Geometry check sheet. Reference: the model listing, model coordinates, mm. Face numbers are marked on the shaded views. A direction names the side the tool comes from. Coordinates: 2 decimals unless noted, no trailing zeros. Loops run counter-clockwise (first coordinate to the right, second up) from the corner with the lowest first, then second, coordinate; pieces in that order, holes last. Notation, with made-up numbers: (50, 49) -> (89, 49) arc R19 ccw to (89, 57) -> close; hole circle Ø9 at (38, 53). An arc over 180 degrees is marked (long way). Answer as a JSON object with one key per item and string values.
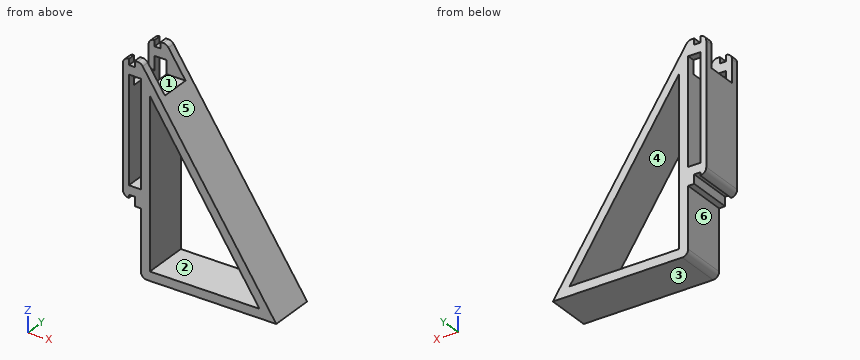
from build123d import *

# Parameters (mm, degrees)
SKETCH2_W               = 4
SKETCH2_H               = 35
BOSS_EXTRUDE1_DEPTH     = 15
CUT_EXTRUDE1_DEPTH      = 87.313382508
CUT_EXTRUDE1_DEPTH_BACK = 15
SKETCH3_W               = 9.5
SKETCH3_H               = 10
FILLET1_R               = 2
FILLET2_R               = 2
FILLET3_R               = 2
FILLET4_R               = 2
FILLET5_R               = 2
FILLET6_R               = 2


with BuildPart() as part:
    # Sketch2 → Boss-Extrude1 (new body)
    with BuildSketch(Plane(origin=(0, 0, 0), x_dir=(1, 0, 0), z_dir=(0, 1, 0))):
        Polygon((0, 0), (0, 2), (2, 2), (2, 0), (4, 0), (49, 68), (4, 68), (4, 46), (2, 46), (2, 43), (0, 43), (0, 44), (-2, 44), (-2, 0), align=None)
        with Locations((2, 22.5)):
            Rectangle(SKETCH2_W, SKETCH2_H, mode=Mode.SUBTRACT)
        Polygon((7, 65), (43.417291153, 65), (7, 9.516238481), align=None, mode=Mode.SUBTRACT)
    extrude(amount=BOSS_EXTRUDE1_DEPTH)

    # Sketch3 → Cut-Extrude1 (cut, two sides: drawn at the far end of the back side and taken through both)
    with BuildSketch(Plane.ZY.offset(2).offset(-CUT_EXTRUDE1_DEPTH_BACK)):
        with Locations((-4.75, 7.5)):
            Rectangle(SKETCH3_W, SKETCH3_H)
    extrude(amount=CUT_EXTRUDE1_DEPTH + CUT_EXTRUDE1_DEPTH_BACK, mode=Mode.SUBTRACT)

    # Fillet1
    fillet1_edges = [part.edges().sort_by_distance(p)[0] for p in [
        (-2, 7.5, -44),
    ]]
    fillet(fillet1_edges, radius=FILLET1_R - 0.0001)  # a hair under: the kernel refuses the full size

    # Fillet2
    fillet2_edges = [part.edges().sort_by_distance(p)[0] for p in [
        (4, 7.5, -68),
    ]]
    fillet(fillet2_edges, radius=FILLET2_R)

    # Fillet3
    fillet3_edges = [part.edges().sort_by_distance(p)[0] for p in [
        (4, 1.25, 0),
    ]]
    fillet(fillet3_edges, radius=FILLET3_R)

    # Fillet4
    fillet4_edges = [part.edges().sort_by_distance(p)[0] for p in [
        (4, 13.75, 0),
    ]]
    fillet(fillet4_edges, radius=FILLET4_R)

    # Fillet5
    fillet5_edges = [part.edges().sort_by_distance(p)[0] for p in [
        (-2, 13.75, 0),
    ]]
    fillet(fillet5_edges, radius=FILLET5_R - 0.0001)  # a hair under: the kernel refuses the full size

    # Fillet6
    fillet6_edges = [part.edges().sort_by_distance(p)[0] for p in [
        (-2, 1.25, 0),
    ]]
    fillet(fillet6_edges, radius=FILLET6_R - 0.0001)  # a hair under: the kernel refuses the full size


solid = part.part
1. Section check D-D, the plane z = -33.5. Record the boundary of the cut face in (x, y), then the cut area to 3 significant figures.
Evaluation:
{"outline": "(-2, 0) -> (0, 0) -> (0, 15) -> (-2, 15) -> close; (4, 0) -> (7, 0) -> (7, 15) -> (4, 15) -> close; (22.74, 0) -> (26.17, 0) -> (26.17, 15) -> (22.74, 15) -> close", "area": "126 mm^2"}
2. Depth check by flat-ended pin: P1, Ø1.6, axis at y = 1, z = -1, coming from the -X side; P2, Ø1.6, axis at x = 2.5, y = 5, coming from the -Z side; P3, Ø5, axis at x = 20.5, y = 7, coming from the +Z side; P4, Ø10.5, axis at x = 7, z = -2.5, coming from the -Y side. Enter the tip coordinate at first touch or a pass-through.
Evaluation:
{"P1": "stops at x = -1.99", "P2": "stops at z = -46", "P3": "stops at z = -21.16", "P4": "stops at y = 0"}
3. Section check C-C, the plane z = -41. Record the boundary of the cut face in (x, y), then the cut area to 3 significant figures.
Evaluation:
{"outline": "(-2, 0) -> (7, 0) -> (7, 15) -> (-2, 15) -> close; (27.66, 0) -> (31.13, 0) -> (31.13, 15) -> (27.66, 15) -> close", "area": "187 mm^2"}
4. Tool access check on the marked faces 1, 2 and 3. Record the directions out of +Z, -Z, +X, -X, +Y, -Y that give a thin tool (end or side, any length) a straight path to the whole face; none if there is none.
Evaluation:
{"face 1": "+Z, +X, -X", "face 2": "+Y, -Y", "face 3": "-Z, +X, -X, +Y, -Y"}
5. Thickness scan on probe 1 along X at (y, z) = (8.5, -20.5); probe 2 along Z at (x, y) = (34, 1); probe 3 along Y at (x, z) = (2, -4). Record the ranges inside material, lowest first. Write a range as from..to.
Evaluation:
{"probe 1": "x = -2..0, 4..7, 14.21..17.57", "probe 2": "z = -68..-65, -50.65..-45.33", "probe 3": "y = 0..2.5, 12.5..15"}
6. Section check B-B, the plane x = 23. Record the boundary of the cut face in (y, z), then the cut area to 3 significant figures.
Evaluation:
{"outline": "(0, -68) -> (15, -68) -> (15, -65) -> (0, -65) -> close; (0, -33.89) -> (15, -33.89) -> (15, -28.71) -> (0, -28.71) -> close", "area": "123 mm^2"}
7. Mould release check, pull along Z, two halves, no side actions. Record for the marked faces 4, 5 and 6: released by +Z, released by -Z, zero draft, split by the parting line, or undercut.
Evaluation:
{"face 4": "undercut", "face 5": "released by +Z", "face 6": "zero draft"}
